Geometry: final body of the model. Coordinates: model frame, mm. Face numbers are marked on the shaded views. A direction names the side the tool comes from. Give positions to 0.01 mm unless a question says otherwise; leave off trailing zeros. Order: outer loops, then holes, each group sorted by start corner. A loop starts at its lowest first (then second) coordinate and runs counter-clockwise, first axis right, second up. Notation, with made-up numbers: (60.25, -20) -> (101.25, -20) arc R15 ccw to (101.25, -4) -> close; hole circle Ø9 at (69.25, 34). An arc over 180 degrees is marked (long way). Write item = value, one per line.
```python
from build123d import *
from build123d.topology import SkipClean

# Parameters (mm, degrees)
SKETCH1_R           = 5
BOSS_EXTRUDE1_DEPTH = 1.6
BOSS_EXTRUDE2_DEPTH = 7.9
CIRPATTERN3_COUNT   = 3
CUT_EXTRUDE2_DEPTH  = 12.240212189
CUT_EXTRUDE3_DEPTH  = 12.310719255
CUT_EXTRUDE4_DEPTH  = 12.10732297


with BuildPart() as part:
    # Sketch1 → Boss-Extrude1 (new body)
    with BuildSketch(Plane(origin=(0, 0, 0), x_dir=(1, 0, 0), z_dir=(0, 1, 0))):
        with Locations(Location((0, 0, 0), (0, 0, 270))):
            Circle(SKETCH1_R)
    extrude(amount=BOSS_EXTRUDE1_DEPTH)

    # Sketch2 → Boss-Extrude2 (add)
    with BuildSketch(Plane(origin=(0, 1.6, 0), x_dir=(1, 0, 0), z_dir=(0, 1, 0))):
        with BuildLine():
            Line((-1.2, 4.85386444), (-1.2, 3.815756806))
            ThreePointArc((-1.2, 3.815756806), (0, 4), (1.2, 3.815756806))
            Line((1.2, 3.815756806), (1.2, 4.85386444))
            ThreePointArc((1.2, 4.85386444), (0, 5), (-1.2, 4.85386444))
        make_face()
    boss_extrude2 = extrude(amount=BOSS_EXTRUDE2_DEPTH)

    # CirPattern3: Boss-Extrude2 ×3 about axis
    cirpattern3_axis = Axis((0, 0, 0), (0, 1, 0))
    for i in range(1, CIRPATTERN3_COUNT):
        add(boss_extrude2.rotate(cirpattern3_axis, i * 360 / CIRPATTERN3_COUNT))

    # Sweep3: sweep along a path in Sketch6
    with SkipClean():  # the faces are left unmerged after this step: merging them gives an invalid solid
        with BuildLine(Plane(origin=(0, 9.5, 0), x_dir=(1, 0, 0), z_dir=(0, 1, 0))) as sweep3_path:
            CenterArc((0, 0), 5, 0, 360)
        # Sketch3 → Sweep3 (sweep)
        with BuildSketch(Plane(origin=(0, 0, 0), x_dir=(0, 0, -1), z_dir=(1, 0, 0))):
            Polygon((5, 9.5), (5.65386444, 8), (4.85386444, 8), (4.85386444, 9.5), align=None)
        sweep(path=sweep3_path.line)
    add(part.part.scale(1), mode=Mode.REPLACE)  # the faces are merged on a copy

    # Sketch7 → Cut-Extrude2 (cut, through all)
    with BuildSketch(Plane(origin=(0, 1.6, 0), x_dir=(1, 0, 0), z_dir=(0, 1, 0))):
        with BuildLine():
            Line((-3.904542328, -0.868647918), (-4.803569911, -1.387701735))
            ThreePointArc((-4.803569911, -1.387701735), (-4.330127019, 2.5), (-1.2, 4.85386444))
            Line((-1.2, 4.85386444), (-1.2, 3.815756806))
            ThreePointArc((-1.2, 3.815756806), (0, 4), (1.2, 3.815756806))
            Line((1.2, 3.815756806), (1.2, 4.85386444))
            ThreePointArc((1.2, 4.85386444), (4.330127019, 2.5), (4.803569911, -1.387701735))
            Line((4.803569911, -1.387701735), (3.904542328, -0.868647918))
            ThreePointArc((3.904542328, -0.868647918), (3.464101615, -2), (2.704542328, -2.947108887))
            Line((2.704542328, -2.947108887), (3.603569911, -3.466162704))
            ThreePointArc((3.603569911, -3.466162704), (0, -5), (-3.603569911, -3.466162704))
            Line((-3.603569911, -3.466162704), (-2.704542328, -2.947108887))
            ThreePointArc((-2.704542328, -2.947108887), (-3.464101615, -2), (-3.904542328, -0.868647918))
        make_face()
    extrude(amount=CUT_EXTRUDE2_DEPTH, mode=Mode.SUBTRACT)

    # Sketch8 → Cut-Extrude3 (cut, through all)
    with BuildSketch(Plane.XZ.offset(-8)):
        with BuildLine():
            Line((-3.603569911, 3.466162704), (-4.184834096, 3.801755738))
            ThreePointArc((-4.184834096, 3.801755738), (0, 5.65386444), (4.184834096, 3.801755738))
            Line((4.184834096, 3.801755738), (3.603569911, 3.466162704))
            ThreePointArc((3.603569911, 3.466162704), (0, 5), (-3.603569911, 3.466162704))
        make_face()
        with BuildLine():
            Line((-5.384834096, 1.723294769), (-4.803569911, 1.387701735))
            ThreePointArc((-4.803569911, 1.387701735), (-4.330127019, -2.5), (-1.2, -4.85386444))
            Line((-1.2, -4.85386444), (-1.2, -5.525050507))
            ThreePointArc((-1.2, -5.525050507), (-4.896390234, -2.82693222), (-5.384834096, 1.723294769))
        make_face()
        with BuildLine():
            Line((1.2, -5.525050507), (1.2, -4.85386444))
            ThreePointArc((1.2, -4.85386444), (4.330127019, -2.5), (4.803569911, 1.387701735))
            Line((4.803569911, 1.387701735), (5.384834096, 1.723294769))
            ThreePointArc((5.384834096, 1.723294769), (4.896390234, -2.82693222), (1.2, -5.525050507))
        make_face()
    extrude(amount=-CUT_EXTRUDE3_DEPTH, mode=Mode.SUBTRACT)

    # Sketch9 → Cut-Extrude4 (cut, through all)
    with BuildSketch(Plane(origin=(0, 1.6, 0), x_dir=(1, 0, 0), z_dir=(0, 1, 0))):
        with BuildLine():
            Line((-1.7, 1.183307578), (-1.7, -1.75))
            ThreePointArc((-1.7, -1.75), (-1.348528137, -2.598528137), (-0.5, -2.95))
            Line((-0.5, -2.95), (0.5, -2.95))
            ThreePointArc((0.5, -2.95), (1.348528137, -2.598528137), (1.7, -1.75))
            Line((1.7, -1.75), (1.7, 1.183307578))
            ThreePointArc((1.7, 1.183307578), (0, 4.516190379), (-1.7, 1.183307578))
        make_face()
    extrude(amount=-CUT_EXTRUDE4_DEPTH, mode=Mode.SUBTRACT)


solid = part.part
```
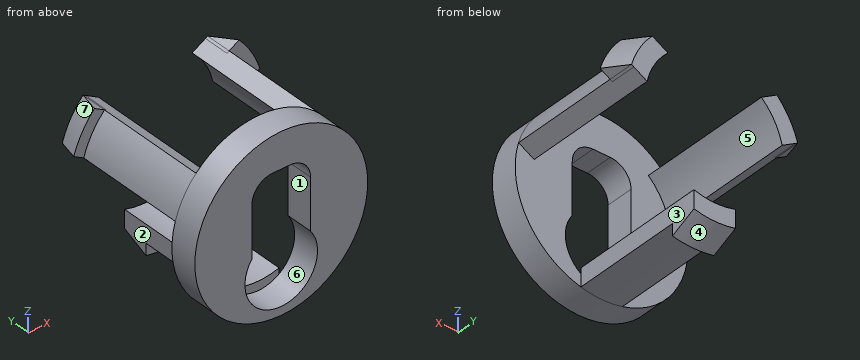
1) Section query B-B (y = 3.75). Output: boundary loops of the cut face in (x, z), plus the area to 3 significant figures.
Check sheet entries:
outline = (-4.8, 1.39) -> (-3.9, 0.87) arc R4 cw to (-2.7, 2.95) -> (-3.6, 3.47) arc R5 ccw to start; (-1.2, -4.85) arc R5 ccw to (1.2, -4.85) -> (1.2, -3.82) arc R4 cw to (-1.2, -3.82) -> close; (2.7, 2.95) arc R4 cw to (3.9, 0.87) -> (4.8, 1.39) arc R5 ccw to (3.6, 3.47) -> close
area = 7.29 mm²
2) Section query C-C (z = -1.75). Output: boundary loops of the cut face in (x, y).
Check sheet entries:
outline = (-4.68, 0) -> (-1.99, 0) -> (-1.99, 1.6) -> (-4.68, 1.6) -> close; (1.99, 0) -> (4.68, 0) -> (4.68, 1.6) -> (1.99, 1.6) -> close
3) First-contact query: P1, Ø3.5, axis at x = 0, z = -2.42, coming from the +Y side; P2, Ø3, axis at x = -1, z = 0, coming from the +Y side; P3, Ø1.8, axis at y = 1, z = 0, coming from the +X side; P4, Ø1.4, axis at y = 7.5, z = -5, coming from the +X side. Flat tips, straight axial feed; report the tip coordinate or a pass-through.
Check sheet entries:
P1 = 9.5
P2 = 1.6
P3 = 5
P4 = 1.2
4) Reachability of the marked faces 1, 2 and 3 from +Z, -Z, +X, -X, +Y, -Y: full face, straight path, thin tool, end or side. Return the list, or none.
Check sheet entries:
face_1 = +Y, -Y
face_2 = +Z, -Z, -X, +Y
face_3 = +Z, -Z, +X, +Y
5) Section query D-D (z = 4). Output: boundary loops of the cut face in (x, y), plus the area to 3 significant figures.
Check sheet entries:
outline = (-3, 0) -> (3, 0) -> (3, 1.6) -> (-3, 1.6) -> close
area = 9.60 mm²
6) Section query A-A (z = 0). Output: boundary loops of the cut face in (x, y), plus the area to 3 significant figures.
Check sheet entries:
outline = (-5, 0) -> (-1.7, 0) -> (-1.7, 1.6) -> (-5, 1.6) -> close; (1.7, 0) -> (5, 0) -> (5, 1.6) -> (1.7, 1.6) -> close
area = 10.6 mm²
7) Line query: line 1 (Z direction, x = 0, y = 0.7); line 2 (X direction, y = 1, z = 0); line 3 (Y direction, x = -1.5, z = -4.5). Output: solid intervals per line, ascending. Write a range as from..to.
Check sheet entries:
line_1 = -5..-4.52, 2.95..5
line_2 = -5..-1.7, 1.7..5
line_3 = 0..1.6
8) Mould query, pull axis X, two halves, no side actions, for the marked faces 4, 5, 6 and 7. Classes: +X half, -X half, draft (parallel to the pull), parting line (faces both ways), or undercut.
Check sheet entries:
face_4 = parting line
face_5 = undercut
face_6 = undercut
face_7 = -X half
